Geometry check sheet. Reference: the model listing, model coordinates, mm. A direction names the side the tool comes from. Round coordinates to 2 decimals unless told otherwise and drop trailing zeros. Write each loop counter-clockwise with the first axis right and the second up, starting at its lowest first coordinate (ties: lowest second). Pieces come first, ordered by that corner, then holes. Notation, with made-up numbers: (70, 1) - (119, 1) arc R7 ccw to (119, 7) - close; hole circle Ø6 at (9, 70.5). An arc over 180 degrees is marked (long way). Return JSON: item names as keys, results as strings. Group by question number.
from build123d import *

# Parameters (mm, degrees)
SKETCH1_R                = 1.5
SKETCH1_R_2              = 2.5
BOSS_EXTRUDE1_DEPTH      = 20
SKETCH2_W                = 8.1
SKETCH2_H                = 20
SKETCH2_W_2              = 5.2
SKETCH2_W_3              = 5.1
CUT_EXTRUDE1_DEPTH       = 20
CUT_EXTRUDE1_DEPTH_BACK  = 20
CUT_EXTRUDE2_DEPTH       = 9
BOSS_EXTRUDE2_DEPTH      = 11.9
SKETCH5_R                = 3
BOSS_EXTRUDE3_DEPTH      = 5
CUT_EXTRUDE6_DEPTH       = 1
SKETCH13_R               = 2.5
CUT_EXTRUDE7_DEPTH       = 4
BOSS_EXTRUDE4_DEPTH      = 3
CUT_EXTRUDE9_DEPTH       = 3
SKETCH17_W               = 9
SKETCH17_H               = 3.569322199
CUT_EXTRUDE11_DEPTH      = 3
SKETCH18_W               = 5.770974844
SKETCH18_H               = 0.772936936
BOSS_EXTRUDE5_DEPTH      = 6.9
BOSS_EXTRUDE5_DEPTH_BACK = 1
SKETCH19_W               = 5.1
SKETCH19_H               = 16.397725614
CUT_EXTRUDE12_DEPTH      = 0.301495
SKETCH20_W               = 5
SKETCH20_H               = 12.419235667
CUT_EXTRUDE13_DEPTH      = 10
BOSS_EXTRUDE6_DEPTH      = 2
SKETCH23_W               = 4.9
SKETCH23_H               = 6
BOSS_EXTRUDE7_DEPTH      = 4
SKETCH22_R               = 1
CUT_EXTRUDE15_DEPTH      = 8
BOSS_EXTRUDE8_DEPTH      = 2
SKETCH14_R               = 1.5
CUT_EXTRUDE8_DEPTH       = 10.1
CUT_EXTRUDE17_DEPTH      = 8.1
CUT_EXTRUDE17_DEPTH_BACK = 2
CUT_EXTRUDE18_DEPTH      = 2
CUT_EXTRUDE20_DEPTH      = 5.2
SKETCH30_W               = 6.9
SKETCH30_H               = 20
CUT_EXTRUDE21_DEPTH      = 0.283797
CUT_EXTRUDE22_REACH      = 91.699
SKETCH31_W               = 2
SKETCH31_H               = 11.022421386
CUT_EXTRUDE23_DEPTH      = 7
CUT_EXTRUDE24_DEPTH      = 21
SKETCH34_W               = 70.65252795
SKETCH34_H               = 74.33474439
CUT_EXTRUDE25_DEPTH      = 21


with BuildPart() as part:
    # Sketch1 → Boss-Extrude1 (new body)
    with BuildSketch(Plane(origin=(0, 0, 0), x_dir=(0, 0, -1), z_dir=(1, 0, 0))):
        with BuildLine():
            ThreePointArc((9.765353557, 20.116545894), (0, 32.270117322), (-9.765353557, 20.116545894))
            ThreePointArc((-9.765353557, 20.116545894), (-5.132645827, -18.047253777), (-7.88740095, -56.392382678))
            ThreePointArc((-7.88740095, -56.392382678), (0, -65.729882678), (7.88740095, -56.392382678))
            ThreePointArc((7.88740095, -56.392382678), (5.132645827, -18.047253777), (9.765353557, 20.116545894))
        make_face()
        with Locations((0, 22.270117322)):
            Circle(SKETCH1_R, mode=Mode.SUBTRACT)
        with Locations((0, -57.729882678)):
            Circle(SKETCH1_R_2, mode=Mode.SUBTRACT)
    extrude(amount=BOSS_EXTRUDE1_DEPTH)

    # Sketch2 → Cut-Extrude1 (cut, two sides)
    with BuildSketch(Plane.XY) as cut_extrude1_sk:
        with Locations((4.05, -55.729882678)):
            Rectangle(SKETCH2_W, SKETCH2_H)
        with Locations((17.4, -55.729882678)):
            Rectangle(SKETCH2_W_2, SKETCH2_H)
        with Locations((5.55, 22.270117322)):
            Rectangle(SKETCH2_W_3, SKETCH2_H)
    extrude(amount=CUT_EXTRUDE1_DEPTH, mode=Mode.SUBTRACT)
    extrude(cut_extrude1_sk.sketch, amount=-CUT_EXTRUDE1_DEPTH_BACK, mode=Mode.SUBTRACT)

    # Sketch3 → Cut-Extrude2 (cut)
    with BuildSketch(Plane.ZY.offset(-8.1)):
        with BuildLine():
            Line((8.5, 22.270117322), (8.5, 40.909533312))
            Line((8.5, 40.909533312), (-17.52872033, 40.909533312))
            Line((-17.52872033, 40.909533312), (-17.52872033, 13.770117322))
            Line((-17.52872033, 13.770117322), (0, 13.770117322))
            ThreePointArc((0, 13.770117322), (6.01040764, 16.259709682), (8.5, 22.270117322))
        make_face()
    extrude(amount=-CUT_EXTRUDE2_DEPTH, mode=Mode.SUBTRACT)

    # Sketch4 → Boss-Extrude2 (add, through all)
    with BuildSketch(Plane.ZY.offset(-8.1)):
        Polygon((8.5, 27.537944199), (8.283796844, 12.741558936), (10.283796844, 12.741558936), (10.283796844, 27.537944199), align=None)
    extrude(amount=-BOSS_EXTRUDE2_DEPTH)

    # Sketch5 → Boss-Extrude3 (add)
    with BuildSketch(Plane.ZY.offset(-8.1)):
        with BuildLine():
            Line((8.145156861, 11.968622), (8.447845456, 23.968622))
            Line((8.447845456, 23.968622), (9.854698466, 23.968622))
            Line((9.854698466, 23.968622), (15.022421386, 23.968622))
            ThreePointArc((15.022421386, 23.968622), (21.022421386, 17.968622), (15.022421386, 11.968622))
            Line((15.022421386, 11.968622), (8.145156861, 11.968622))
        make_face()
        with Locations((15.022421386, 17.968622)):
            Circle(SKETCH5_R, mode=Mode.SUBTRACT)
    extrude(amount=-BOSS_EXTRUDE3_DEPTH)

    # Sketch12 → Cut-Extrude6 (cut)
    with BuildSketch(Plane(origin=(13.1, 0, 0), x_dir=(0, 0, -1), z_dir=(1, 0, 0))):
        Polygon((-13.902900694, 14.968622), (-13.902900694, 12.968622), (-15.902900694, 12.968622), (-15.902900694, 14.968622), (-15.902900694, 15.294296094), (-13.902900694, 15.294296094), align=None)
    extrude(amount=-CUT_EXTRUDE6_DEPTH, mode=Mode.SUBTRACT)

    # Sketch13 → Cut-Extrude7 (cut)
    with BuildSketch(Plane.ZY.offset(-17.1)):
        with Locations((0, 22.270117322)):
            Circle(SKETCH13_R)
    extrude(amount=-CUT_EXTRUDE7_DEPTH, mode=Mode.SUBTRACT)

    # Sketch15 → Boss-Extrude4 (add)
    with BuildSketch(Plane.ZY):
        Polygon((10, 22.270117322), (10, 11.968622), (8.145156861, 11.968622), (7.595672539, 11.968622), align=None)
    extrude(amount=-BOSS_EXTRUDE4_DEPTH)

    # Sketch16 → Cut-Extrude9 (cut)
    with BuildSketch(Plane(origin=(20, 0, 0), x_dir=(0, 0, -1), z_dir=(1, 0, 0))):
        with BuildLine():
            Line((-10.283796844, 23.968622), (-9.854698466, 23.968622))
            ThreePointArc((-9.854698466, 23.968622), (-9.349264901, 25.818531871), (-8.5, 27.537944199))
            Line((-8.5, 27.537944199), (-10.283796844, 27.537944199))
            Line((-10.283796844, 27.537944199), (-10.283796844, 23.968622))
        make_face()
    extrude(amount=-CUT_EXTRUDE9_DEPTH, mode=Mode.SUBTRACT)

    # Sketch17 → Cut-Extrude11 (cut)
    with BuildSketch(Plane.XY.offset(10.283796844)):
        with Locations((12.6, 25.7532831)):
            Rectangle(SKETCH17_W, SKETCH17_H)
    extrude(amount=-CUT_EXTRUDE11_DEPTH, mode=Mode.SUBTRACT)

    # Sketch18 → Boss-Extrude5 (add, two sides)
    with BuildSketch(Plane(origin=(13.1, 0, 0), x_dir=(0, 0, -1), z_dir=(1, 0, 0))) as boss_extrude5_sk:
        with Locations((-7.398309422, 12.355090468)):
            Rectangle(SKETCH18_W, SKETCH18_H)
    extrude(amount=BOSS_EXTRUDE5_DEPTH)
    extrude(boss_extrude5_sk.sketch, amount=-BOSS_EXTRUDE5_DEPTH_BACK)

    # Sketch19 → Cut-Extrude12 (cut)
    with BuildSketch(Plane(origin=(0, 12.270117322, 0), x_dir=(1, 0, 0), z_dir=(0, 1, 0))):
        with Locations((5.55, 0)):
            Rectangle(SKETCH19_W, SKETCH19_H)
    extrude(amount=-CUT_EXTRUDE12_DEPTH, mode=Mode.SUBTRACT)

    # Sketch20 → Cut-Extrude13 (cut)
    with BuildSketch(Plane.ZY.offset(-17.1)):
        with Locations((0, 28.479735156)):
            Rectangle(SKETCH20_W, SKETCH20_H)
    extrude(amount=-CUT_EXTRUDE13_DEPTH, mode=Mode.SUBTRACT)

    # Sketch21 → Boss-Extrude6 (add)
    with BuildSketch(Plane.ZY.offset(-17.1)):
        with BuildLine():
            Line((-8.473151119, 13.770117322), (0.278481736, 12.273995678))
            ThreePointArc((0.278481736, 12.273995678), (9.936881703, 21.148341047), (2.5, 31.952575688))
            Line((2.5, 31.952575688), (2.5, 22.270117322))
            ThreePointArc((2.5, 22.270117322), (0, 19.770117322), (-2.5, 22.270117322))
            Line((-2.5, 22.270117322), (-2.5, 31.952575688))
            ThreePointArc((-2.5, 31.952575688), (-8.522477621, 27.501501002), (-9.765353557, 20.116545894))
            ThreePointArc((-9.765353557, 20.116545894), (-9.093560923, 16.948562662), (-8.473151119, 13.770117322))
        make_face()
    extrude(amount=BOSS_EXTRUDE6_DEPTH)

    # Sketch23 → Boss-Extrude7 (add)
    with BuildSketch(Plane.XY.offset(10.283796844)):
        with Locations((17.55, 26.968622)):
            Rectangle(SKETCH23_W, SKETCH23_H)
    extrude(amount=-BOSS_EXTRUDE7_DEPTH)

    # Sketch22 → Cut-Extrude15 (cut)
    with BuildSketch(Plane.XY.offset(10.283796844)):
        with Locations((17.55, 26.870117322)):
            Circle(SKETCH22_R)
    extrude(amount=-CUT_EXTRUDE15_DEPTH, mode=Mode.SUBTRACT)

    # Sketch24 → Boss-Extrude8 (add)
    with BuildSketch(Plane.ZY.offset(-8.1)):
        with BuildLine():
            Line((5.147845456, 19.737443909), (5.147845456, 15.506265819))
            Line((5.147845456, 15.506265819), (8.447845456, 15.506265819))
            Line((8.447845456, 15.506265819), (8.447845456, 23.968622))
            add(Edge.make_bspline(
                [(8.447845456, 23.968622), (5.147845456, 23.968622), (5.147845456, 19.737443909)],
                knots=[3.141592654, 3.141592654, 3.141592654, 4.71238898, 4.71238898, 4.71238898], degree=2, weights=[1, 0.707106781, 1]))
        make_face()
    extrude(amount=-BOSS_EXTRUDE8_DEPTH)

    # Sketch14 → Cut-Extrude8 (cut)
    with BuildSketch(Plane.ZY):
        with Locations((7.532575614, 18.331804915)):
            Circle(SKETCH14_R)
    extrude(amount=-CUT_EXTRUDE8_DEPTH, mode=Mode.SUBTRACT)

    # Sketch25 → Cut-Extrude17 (cut, two sides)
    with BuildSketch(Plane.ZY.offset(-8.1)) as cut_extrude17_sk:
        with BuildLine():
            Line((12, -45.729882678), (8.346153846, -36.960651908))
            ThreePointArc((8.346153846, -36.960651908), (6.973852263, -42.37911752), (2.5, -45.729882678))
            Line((2.5, -45.729882678), (2.5, -53.227383372))
            ThreePointArc((2.5, -53.227383372), (0, -62.879882678), (-2.5, -53.227383372))
            Line((-2.5, -53.227383372), (-2.5, -45.729882678))
            ThreePointArc((-2.5, -45.729882678), (-6.973852263, -42.37911752), (-8.346153846, -36.960651908))
            Line((-8.346153846, -36.960651908), (-12, -45.729882678))
            Line((-12, -45.729882678), (-12, -57.729882678))
            ThreePointArc((-12, -57.729882678), (0, -69.729882678), (12, -57.729882678))
            Line((12, -57.729882678), (12, -45.729882678))
        make_face()
    extrude(amount=CUT_EXTRUDE17_DEPTH, mode=Mode.SUBTRACT)
    extrude(cut_extrude17_sk.sketch, amount=-CUT_EXTRUDE17_DEPTH_BACK, mode=Mode.SUBTRACT)

    # Sketch26 → Cut-Extrude18 (cut)
    with BuildSketch(Plane(origin=(20, 0, 0), x_dir=(0, 0, -1), z_dir=(1, 0, 0))):
        with BuildLine():
            Line((-7.209968303, 15.085404497), (-10.283796844, 15.085404497))
            Line((-10.283796844, 15.085404497), (-10.283796844, 17.085404497))
            Line((-10.283796844, 17.085404497), (-7.209968303, 17.085404497))
            ThreePointArc((-7.209968303, 17.085404497), (-4.010444351, 15.949526558), (-2.243391617, 13.050441039))
            ThreePointArc((-2.243391617, 13.050441039), (0.649659998, -12.257973546), (0.397031114, -37.729953741))
            Line((0.397031114, -37.729953741), (-1.608183929, -37.729953741))
            ThreePointArc((-1.608183929, -37.729953741), (-1.343036313, -12.450773719), (-4.206611504, 12.667092093))
            ThreePointArc((-4.206611504, 12.667092093), (-5.281990934, 14.405678614), (-7.209968303, 15.085404497))
        make_face()
    extrude(amount=-CUT_EXTRUDE18_DEPTH, mode=Mode.SUBTRACT)

    # Sketch29 → Cut-Extrude20 (cut)
    with BuildSketch(Plane(origin=(20, 0, 0), x_dir=(0, 0, -1), z_dir=(1, 0, 0))):
        with BuildLine():
            Line((8, -37.729882678), (8.140336581, -37.729882678))
            Line((8.140336581, -37.729882678), (8.140336581, -45.937498976))
            Line((8.140336581, -45.937498976), (-15.754893946, -45.937498976))
            Line((-15.754893946, -45.937498976), (-15.754893946, -37.729882678))
            Line((-15.754893946, -37.729882678), (-8, -37.729882678))
            ThreePointArc((-8, -37.729882678), (0, -45.729882678), (8, -37.729882678))
        make_face()
    extrude(amount=-CUT_EXTRUDE20_DEPTH, mode=Mode.SUBTRACT)

    # Sketch30 → Cut-Extrude21 (cut)
    with BuildSketch(Plane.XY.offset(10.283796844)):
        with Locations((16.55, 21.968622)):
            Rectangle(SKETCH30_W, SKETCH30_H)
    extrude(amount=-CUT_EXTRUDE21_DEPTH, mode=Mode.SUBTRACT)

    # Sketch31 → Cut-Extrude22 (cut, up to next)
    with BuildSketch(Plane(origin=(0, 23.968622, 0), x_dir=(1, 0, 0), z_dir=(0, 1, 0)), mode=Mode.PRIVATE) as cut_extrude22_sk1:
        with Locations((9.1, -15.511210693)):
            Rectangle(SKETCH31_W, SKETCH31_H)
    cut_extrude22_tool1 = extrude(cut_extrude22_sk1.sketch, amount=-CUT_EXTRUDE22_REACH, mode=Mode.PRIVATE) & part.part
    add(cut_extrude22_tool1.solids().sort_by_distance((9.1, 23.968622, 15.511211))[0], mode=Mode.SUBTRACT)

    # Sketch32 → Cut-Extrude23 (cut)
    with BuildSketch(Plane.ZY.offset(-8.1)):
        Polygon((-8.473151119, 13.770117322), (-8.473151119, 5.401068454), (5.147845456, 15.506265819), align=None)
    extrude(amount=-CUT_EXTRUDE23_DEPTH, mode=Mode.SUBTRACT)

    # Sketch33 → Cut-Extrude24 (cut, through all)
    with BuildSketch(Plane(origin=(20, 0, 0), x_dir=(0, 0, -1), z_dir=(1, 0, 0))):
        Polygon((-9.30475326, -22.954882678), (-9.30475326, -27.954882678), (8.892389241, -27.954882678), (8.892389241, -22.954882678), (8.892389241, -17.954882678), (-9.30475326, -17.954882678), align=None)
    extrude(amount=-CUT_EXTRUDE24_DEPTH, mode=Mode.SUBTRACT)

    # Sketch34 → Cut-Extrude25 (cut, through all)
    with BuildSketch(Plane(origin=(20, 0, 0), x_dir=(0, 0, -1), z_dir=(1, 0, 0))):
        with Locations((-4.594652679, 17.444902541)):
            Rectangle(SKETCH34_W, SKETCH34_H)
    extrude(amount=-CUT_EXTRUDE25_DEPTH, mode=Mode.SUBTRACT)


solid = part.part
1. Section check C-C (z = -3). Enter the section's corners in (x, y).
2. Section check D-D (y = -34.5). Enter the section's corners in (x, z).
3. Section check A-A (z = 0). Enter the section's corners in (x, y).
4. Section check B-B (x = 5.5). Enter the section's corners in (y, z).
5. Material ranges on line 1 along Y through (x, z) = (11, 0); line 2 along X through (y, z) = (-59.5, -2.25); line 3 along X through (y, z) = (-56, -5.75), recorded low to high.
6. Tool access check on faces 1 (the face through (9, -50, -2.5)), 2 (the face through (4, -45.73, 0)), 3 (the face through (19.014, -32.914, 1.316)), 4 (the face through (10.1, -52, 3)). Record the directions out of +Z, -Z, +X, -X, +Y, -Y that give a thin tool (end or side, any length) a straight path to the whole face; none if there is none.
7. Depth check by flat-ended pin: pin 1 Ø2 at (x, y) = (9, -48.5) entering from -Z; pin 2 Ø5 at (y, z) = (-58.5, -0.5) entering from -X; pin 3 Ø3 at (x, y) = (10.5, -32) entering from -Z. Enter the tip coordinate at first touch or a pass-through.
8. Mould release check, pull along Z, two halves, no side actions. Record for faces 5 (the face through (5.12, -44.84, -4.44)), 6 (the face through (9, -49, 2.5)), 7 (the face through (18, -33, 0)): pulls with the +Z half, pulls with the -Z half, needs draft (parallel to the pull), parting line crosses it, or undercut.
Result sheet:
{
 "1": {"outline": "(0, -45.56) - (10.1, -45.56) - (10.1, -53.54) - (8.1, -53.54) - (8.1, -61.92) - (10.1, -61.92) - (10.1, -65.15) - (14.8, -65.15) - (14.8, -45.15) - (20, -45.15) - (20, -27.95) - (0, -27.95) - close"},
 "2": {"outline": "(0, -5.41) - (20, -5.41) - (20, -0.6) - (18, -0.6) - (18, 1.4) - (20, 1.4) - (20, 5.41) - (0, 5.41) - close"},
 "3": {"outline": "(0, -45.73) - (8.1, -45.73) - (8.1, -55.23) - (14.8, -55.23) - (14.8, -45.73) - (20, -45.73) - (20, -37.73) - (18, -37.73) - (18, -27.95) - (0, -27.95) - close; (8.1, -62.88) - (10.1, -62.88) - (10.1, -65.73) - (14.8, -65.73) - (14.8, -60.23) - (8.1, -60.23) - close"},
 "4": {"outline": "(-45.73, -2.5) arc R8.38 ccw to (-43.45, -6.13) arc R200 cw to (-27.95, -5.13) - (-27.95, 5.13) arc R200 cw to (-43.45, 6.13) arc R8.38 ccw to (-45.73, 2.5) - close"},
 "5": {"line 1": "y = -65.73 to -60.23, -55.23 to -27.95", "line 2": "x = 8.1 to 14.8", "line 3": "x = 10.1 to 14.8"},
 "6": {"face 1": "-Z, -X", "face 2": "+Z, -Z, -X, -Y", "face 3": "+X", "face 4": "-X"},
 "7": {"pin 1": "stops at z = -2.5", "pin 2": "stops at x = 8.1", "pin 3": "stops at z = -5.35"},
 "8": {"face 5": "pulls with the -Z half", "face 6": "pulls with the +Z half", "face 7": "undercut"}
}
